Geometry: final body of the model. Coordinates: model frame, mm. Round coordinates to 2 decimals unless told otherwise and drop trailing zeros. Write each loop counter-clockwise with the first axis right and the second up, starting at its lowest first coordinate (ties: lowest second). Pieces come first, ordered by that corner, then holes. Notation, with made-up numbers: (74, 8.5) -> (85, 8.5) arc R24 cw to (85, 24.5) -> close; hole circle Ø9 at (-30.5, -35.5). An arc over 180 degrees is marked (long way). Use one line per item in the form item = value. Start each with the question number.
1. Cut plane B-B, the plane z = 3.25. State how many separate pieces and enclosed holes the cut face has, plus the area to 3 significant figures.
2. Cut plane A-A, the plane x = 117.5. Return the cut outline in (y, z), plus the area to 3 significant figures.
3. Line query: L1, parallel to Y at x = 15, z = 1.25; L2, parallel to X at y = -150, z = 2.75; L3, parallel to Y at x = -46, z = 3. Output: solid intervals per line, ascending.
4. Pin query (flat end, axial travel): pin 1 Ø9 at (x, y) = (-63.5, -3.5) entering from -Z. Return the tip coordinate at first contact, or that it passes through.
```python
from build123d import *

# Parameters (mm, degrees)
F0_W      = 600
F0_H      = 450
F1_DEPTH  = 10
F2_R      = 3.5
F3_DEPTH  = 10
F4_W      = 43
F4_H      = 43
F4_R      = 1.5
F5_DEPTH  = 5
F6_DEPTH  = 10
F4_W_2    = 150
F4_H_2    = 20
F7_DEPTH  = 10
F8_DEPTH  = 10
F9_DEPTH  = 10
F10_DEPTH = 10


with BuildPart() as f1:
    # F0 (on Top) → F1 (new body)
    with BuildSketch(Plane.XY):
        Rectangle(F0_W, F0_H)
    extrude(amount=F1_DEPTH)

    # F2 (on face) → F3 (cut)
    with BuildSketch(Plane.XY.offset(10)):
        with Locations((-63.5, 206.5)):
            Circle(F2_R)
        with Locations((-63.5, 191.5)):
            Circle(F2_R)
        with Locations((-63.5, 176.5)):
            Circle(F2_R)
        with Locations((-63.5, 161.5)):
            Circle(F2_R)
        with Locations((-63.5, 146.5)):
            Circle(F2_R)
        with Locations((-63.5, 131.5)):
            Circle(F2_R)
        with Locations((-63.5, 116.5)):
            Circle(F2_R)
        with Locations((-63.5, 101.5)):
            Circle(F2_R)
        with Locations((-63.5, 86.5)):
            Circle(F2_R)
        with Locations((-63.5, 71.5)):
            Circle(F2_R)
        with Locations((-63.5, 56.5)):
            Circle(F2_R)
        with Locations((-63.5, 41.5)):
            Circle(F2_R)
        with Locations((-63.5, 26.5)):
            Circle(F2_R)
        with Locations((-63.5, 11.5)):
            Circle(F2_R)
        with Locations((-63.5, -3.5)):
            Circle(F2_R)
        with Locations((-63.5, -18.5)):
            Circle(F2_R)
        with Locations((-63.5, -33.5)):
            Circle(F2_R)
        with Locations((-63.5, -48.5)):
            Circle(F2_R)
        with Locations((-63.5, -63.5)):
            Circle(F2_R)
        with Locations((-63.5, -78.5)):
            Circle(F2_R)
        with Locations((63.5, 191.5)):
            Circle(F2_R)
        with Locations((63.5, 86.5)):
            Circle(F2_R)
        with Locations((63.5, 41.5)):
            Circle(F2_R)
        with Locations((63.5, 26.5)):
            Circle(F2_R)
        with Locations((63.5, 101.5)):
            Circle(F2_R)
        with Locations((63.5, -18.5)):
            Circle(F2_R)
        with Locations((63.5, 131.5)):
            Circle(F2_R)
        with Locations((63.5, -63.5)):
            Circle(F2_R)
        with Locations((63.5, 71.5)):
            Circle(F2_R)
        with Locations((63.5, 161.5)):
            Circle(F2_R)
        with Locations((63.5, 176.5)):
            Circle(F2_R)
        with Locations((63.5, -48.5)):
            Circle(F2_R)
        with Locations((63.5, 11.5)):
            Circle(F2_R)
        with Locations((63.5, -78.5)):
            Circle(F2_R)
        with Locations((63.5, -33.5)):
            Circle(F2_R)
        with Locations((63.5, 146.5)):
            Circle(F2_R)
        with Locations((63.5, -3.5)):
            Circle(F2_R)
        with Locations((63.5, 116.5)):
            Circle(F2_R)
        with Locations((63.5, 56.5)):
            Circle(F2_R)
        with Locations((63.5, 206.5)):
            Circle(F2_R)
    extrude(amount=-F3_DEPTH, mode=Mode.SUBTRACT)

    # F4 (on face) → F5 (cut)
    with BuildSketch(Plane.XY.offset(10)):
        with Locations((0, -193.5)):
            Rectangle(F4_W, F4_H)
        with Locations((-15.5, -209)):
            Circle(F4_R, mode=Mode.SUBTRACT)
        with Locations((-15.5, -178)):
            Circle(F4_R, mode=Mode.SUBTRACT)
        with Locations((15.5, -209)):
            Circle(F4_R, mode=Mode.SUBTRACT)
        with Locations((15.5, -178)):
            Circle(F4_R, mode=Mode.SUBTRACT)
    extrude(amount=-F5_DEPTH, mode=Mode.SUBTRACT)

    # F6 (cut): faces of the model
    f6_faces = [f1.faces().sort_by_distance(p)[0] for p in [
        (15.5, -209, 10),
        (15.5, -178, 10),
        (-15.5, -178, 10),
        (-15.5, -209, 10),
    ]]
    extrude(f6_faces, amount=-F6_DEPTH, mode=Mode.SUBTRACT)

    # F4 (on face) → F7 (cut)
    with BuildSketch(Plane.XY.offset(10)):
        with Locations((0, -152)):
            Rectangle(F4_W_2, F4_H_2)
    extrude(amount=-F7_DEPTH, mode=Mode.SUBTRACT)

    # F4 (on face) → F8 (cut)
    with BuildSketch(Plane.XY.offset(10)):
        with BuildLine():
            Line((227.5, -157), (82.5, -157))
            ThreePointArc((82.5, -157), (80, -159.5), (82.5, -162))
            Line((82.5, -162), (227.5, -162))
            ThreePointArc((227.5, -162), (230, -159.5), (227.5, -157))
        make_face()
    extrude(amount=-F8_DEPTH, mode=Mode.SUBTRACT)

    # F4 (on face) → F9 (cut)
    with BuildSketch(Plane.XY.offset(10)):
        with BuildLine():
            ThreePointArc((83, -148), (81, -150), (83, -152))
            Line((83, -152), (228, -152))
            ThreePointArc((228, -152), (230, -150), (228, -148))
            Line((228, -148), (83, -148))
        make_face()
    extrude(amount=-F9_DEPTH, mode=Mode.SUBTRACT)

    # F2 (on face) → F10 (cut)
    with BuildSketch(Plane.XY.offset(10)):
        with Locations((-63.5, 206.5)):
            Circle(F2_R)
        with Locations((-63.5, 191.5)):
            Circle(F2_R)
        with Locations((-63.5, 176.5)):
            Circle(F2_R)
        with Locations((-63.5, 161.5)):
            Circle(F2_R)
        with Locations((-63.5, 146.5)):
            Circle(F2_R)
        with Locations((-63.5, 131.5)):
            Circle(F2_R)
        with Locations((-63.5, 116.5)):
            Circle(F2_R)
        with Locations((-63.5, 101.5)):
            Circle(F2_R)
        with Locations((-63.5, 86.5)):
            Circle(F2_R)
        with Locations((-63.5, 71.5)):
            Circle(F2_R)
        with Locations((-63.5, 56.5)):
            Circle(F2_R)
        with Locations((-63.5, 41.5)):
            Circle(F2_R)
        with Locations((-63.5, 26.5)):
            Circle(F2_R)
        with Locations((-63.5, 11.5)):
            Circle(F2_R)
        with Locations((-63.5, -3.5)):
            Circle(F2_R)
        with Locations((-63.5, -18.5)):
            Circle(F2_R)
        with Locations((-63.5, -33.5)):
            Circle(F2_R)
        with Locations((-63.5, -48.5)):
            Circle(F2_R)
        with Locations((-63.5, -63.5)):
            Circle(F2_R)
        with Locations((-63.5, -78.5)):
            Circle(F2_R)
        with Locations((63.5, 191.5)):
            Circle(F2_R)
        with Locations((63.5, 86.5)):
            Circle(F2_R)
        with Locations((63.5, 41.5)):
            Circle(F2_R)
        with Locations((63.5, 26.5)):
            Circle(F2_R)
        with Locations((63.5, 101.5)):
            Circle(F2_R)
        with Locations((63.5, -18.5)):
            Circle(F2_R)
        with Locations((63.5, 131.5)):
            Circle(F2_R)
        with Locations((63.5, -63.5)):
            Circle(F2_R)
        with Locations((63.5, 71.5)):
            Circle(F2_R)
        with Locations((63.5, 161.5)):
            Circle(F2_R)
        with Locations((63.5, 176.5)):
            Circle(F2_R)
        with Locations((63.5, -48.5)):
            Circle(F2_R)
        with Locations((63.5, 11.5)):
            Circle(F2_R)
        with Locations((63.5, -78.5)):
            Circle(F2_R)
        with Locations((63.5, -33.5)):
            Circle(F2_R)
        with Locations((63.5, 146.5)):
            Circle(F2_R)
        with Locations((63.5, -3.5)):
            Circle(F2_R)
        with Locations((63.5, 116.5)):
            Circle(F2_R)
        with Locations((63.5, 56.5)):
            Circle(F2_R)
        with Locations((63.5, 206.5)):
            Circle(F2_R)
    extrude(amount=-F10_DEPTH, mode=Mode.SUBTRACT)


solid = f1.part
```
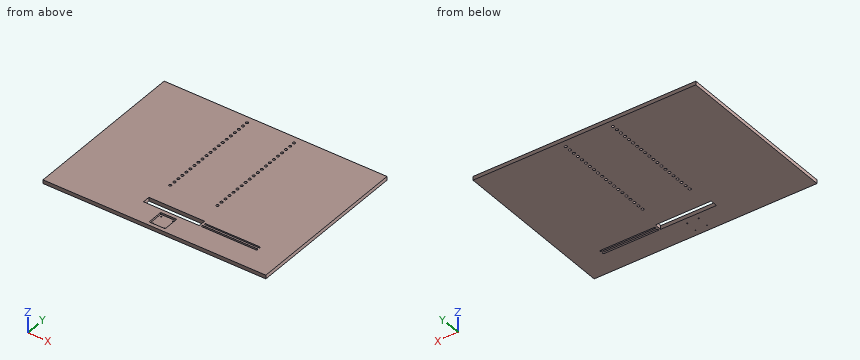
Outcome:
q1.separate_pieces = 1
q1.enclosed_holes = 47
q1.area = 264,000 mm^2
q2.outline = (-225, 0) -> (-162, 0) -> (-162, 10) -> (-225, 10) -> close; (-157, 0) -> (-152, 0) -> (-152, 10) -> (-157, 10) -> close; (-148, 0) -> (225, 0) -> (225, 10) -> (-148, 10) -> close
q2.area = 4,410 mm^2
q3.L1 = -225 to -210.41, -207.59 to -179.41, -176.59 to -162, -142 to 225
q3.L2 = -300 to -75, 75 to 81, 230 to 300
q3.L3 = -225 to -162, -142 to 225
q4.pin_1 = 0
